Input: dimensioned drawing with shaded views. Units: mm. Origin: part minimum x, y, z. A direction names the side the tool comes from. Coordinates: 2 decimals unless noted, no trailing zeros. Loops run counter-clockwise (first coordinate to the right, second up) from the corner with the lowest first, then second, coordinate; pieces in that order, holes last.
(1) Section C-C, the plane y = 2. Return loops of the section in (x, z).
(2) Section D-D, the plane x = 11.75. Return loops of the section in (y, z), then the cut area to 3 significant figures.
(3) Contact query for flat-ended pins moving along their axis: P1, Ø1, axis at x = 9, z = 3.5, coming from the -Y side; P2, Ø1.1, axis at y = 7.5, z = 3.5, coming from the -X side; P3, Ø0.5, axis at x = 7, y = 7.5, coming from the -Z side; P4, Ø1, axis at y = 1, z = 7, coming from the +X side. Output: stop coordinate, or through.
(4) Set-up query: the marked faces 1 and 2. Return all of +Z, -Z, +X, -X, +Y, -Y with unobstructed straight access to the full face (end or side cutting, diameter ignored); none if empty.
(5) Section B-B, the plane z = 6.5. Return loops of the section in (x, y), then the cut area to 3 significant figures.
(6) Line query: L1, parallel to X at y = 7.75, z = 1.75; L2, parallel to Y at x = 1.25, z = 6.75; L3, parallel to X at y = 5.25, z = 4. Output: solid intervals per line, ascending.
(7) Section A-A, the plane z = 3. Return loops of the section in (x, y), then the cut area to 3 significant figures.
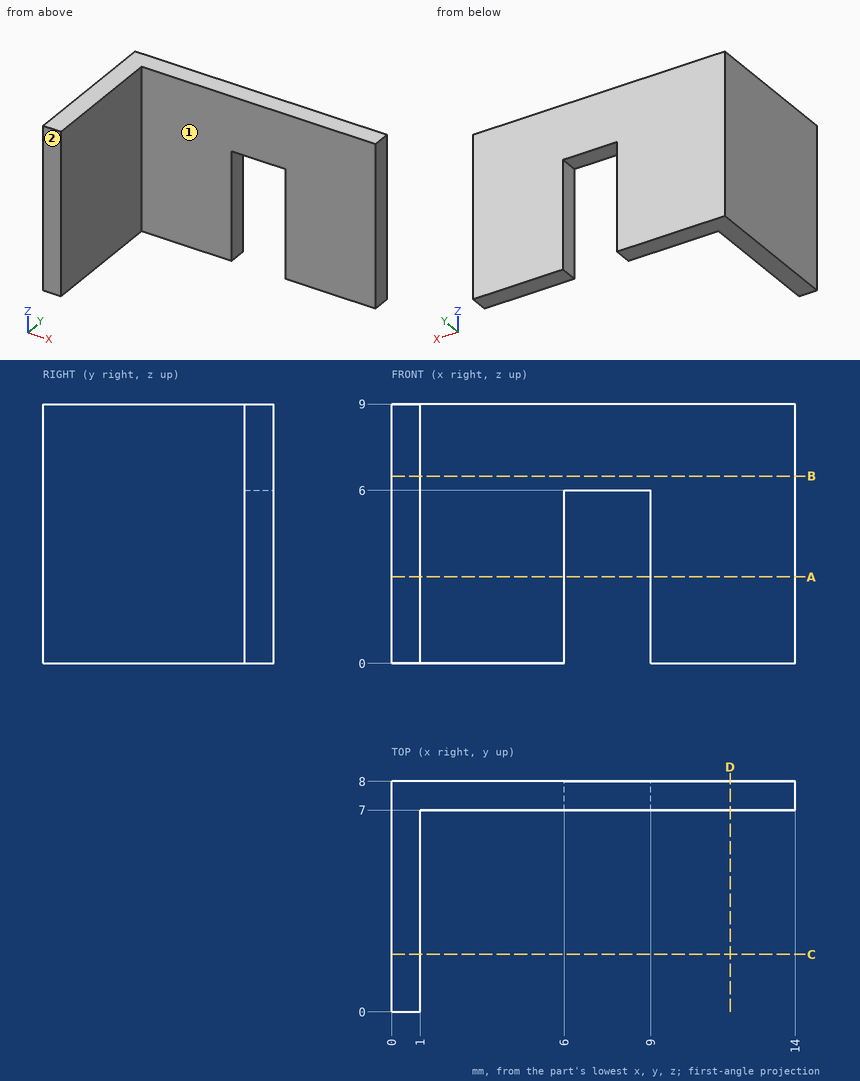
Report:
1. outline: (0, 0) - (1, 0) - (1, 9) - (0, 9) - close
2. outline: (7, 0) - (8, 0) - (8, 9) - (7, 9) - close
2. area: 9.00 mm2
3. P1: stops at y = 7
3. P2: stops at x = 0
3. P3: stops at z = 6
3. P4: stops at x = 1
4. face 1: +Z, -Z, +X, -Y
4. face 2: +Z, -Z, +X, -X, -Y
5. outline: (0, 0) - (1, 0) - (1, 7) - (14, 7) - (14, 8) - (0, 8) - close
5. area: 21.0 mm2
6. L1: x = 0 to 6, 9 to 14
6. L2: y = 7 to 8
6. L3: x = 0 to 1
7. outline: (0, 0) - (1, 0) - (1, 7) - (6, 7) - (6, 8) - (0, 8) - close; (9, 7) - (14, 7) - (14, 8) - (9, 8) - close
7. area: 18.0 mm2
